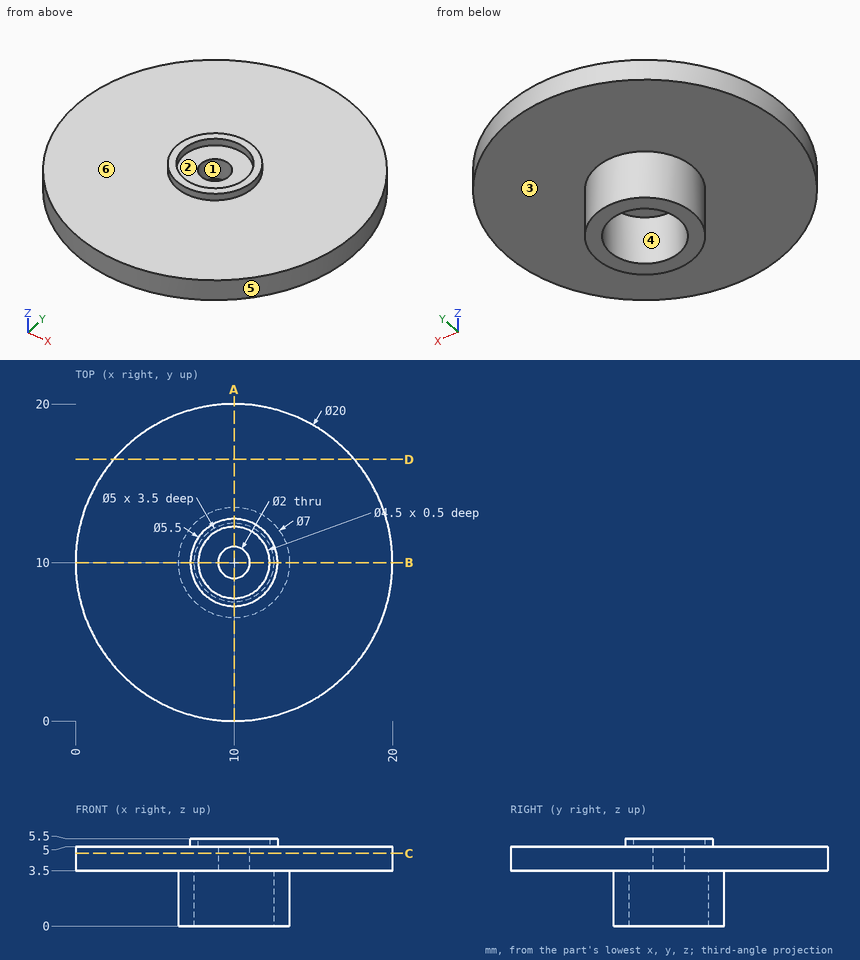
The figure shows three views and two pictorial views of one solid part (mm, origin at its lowest corner). Answer the questions. A direction names the side the tool comes from. Coordinates: 2 decimals unless noted, no trailing zeros. Order: outer loops, then holes, each group sorted by start corner. A loop starts at its lowest first (then second) coordinate and runs counter-clockwise, first axis right, second up.
Q1. A cutting plane is placed at D-D, the plane y = 16.5. Write down the section's boundary in (x, z).
Q2. Given P1, Ø8, axis at x = 5.5, y = 17.5, coming from the -Z side; P2, Ø1.5, axis at y = 9, z = 5, coming from the +X side, each flat-ended and moving along its own axis, determine where each tip first touches the part or whether it passes through.
Q3. A cutting plane is placed at C-C, the plane z = 4.6. Write down the section's boundary in (x, y).
Q4. A cutting plane is placed at A-A, the plane x = 10. Write down the section's boundary in (y, z).
Q5. For a pull along X with two mould halves and no side action, classify the marked faces 4, 5 and 6 as pulls with the +X half, pulls with the -X half, needs draft (parallel to the pull), parting line crosses it, or undercut.
Q6. Which of the six approach directions +Z, -Z, +X, -X, +Y, -Y give full straight-line access (tool end or side, diameter ignored) to the marked faces 1, 2 and 3?
Q7. Consider line 1 (X direction, y = 10, z = 0.9); line 2 (X direction, y = 10, z = 5.45). Determine where each line is inside the solid, lowest interval first.
Answers follow:
1. outline: (2.4, 3.5) - (17.6, 3.5) - (17.6, 5) - (2.4, 5) - close
2. P1: stops at z = 3.5
2. P2: stops at x = 20
3. outline: circle Ø20 at (10, 10); hole circle Ø2 at (10, 10)
4. outline: (0, 3.5) - (6.5, 3.5) - (6.5, 0) - (7.5, 0) - (7.5, 3.5) - (9, 3.5) - (9, 5) - (7.75, 5) - (7.75, 5.5) - (7.25, 5.5) - (7.25, 5) - (0, 5) - close; (11, 3.5) - (12.5, 3.5) - (12.5, 0) - (13.5, 0) - (13.5, 3.5) - (20, 3.5) - (20, 5) - (12.75, 5) - (12.75, 5.5) - (12.25, 5.5) - (12.25, 5) - (11, 5) - close
5. face 4: undercut
5. face 5: parting line crosses it
5. face 6: needs draft
6. face 1: +Z, -Z
6. face 2: +Z
6. face 3: -Z
7. line 1: x = 6.5 to 7.5, 12.5 to 13.5
7. line 2: x = 7.25 to 7.75, 12.25 to 12.75
